Could you check a few things on this model? Use its own coordinates, in mm. A direction names the side the tool comes from. Give positions to 0.01 mm unless a question says otherwise; leave off trailing zeros. Write each loop counter-clockwise with the first axis right and the second up, starting at its lowest first coordinate (ties: lowest second). Pieces come first, ordered by that corner, then holes. Notation, with made-up numbers: (86, -5.5) - (122, -5.5) arc R28 cw to (122, 31.5) - close; hole circle Ø11 at (32, 35). An arc over 180 degrees is marked (long way). Answer as CSV lines item,"result". Start each with the question number.
Q1. If I drill on line 1 along Y through (x, z) = (-65, 2.8); line 2 along Y through (x, z) = (-33.5, 1.8), over which ranges is the centre line in solid material (lowest first)?
Q2. Imagine slicing it at B-B on x = -64. List the corners of the cut face in (y, z) for me.
Q3. Will this pin go through, and if not, where does the flat tip stop? pin 1 Ø1.5 at (y, z) = (-73.5, 1.5) entering from -X.
Q4. We'd pull the mould along X, two halves only. Please class faces 3 (the face through (0, -41, 1)), 4 (the face through (-35.356, -5.994, 1.479)), 5 (the face through (-6.6, -19.1, 0)): pulls with the +X half, pulls with the -X half, needs draft (parallel to the pull), parting line crosses it, or undercut.
Q5. Imagine slicing it at A-A on z = 1.6. List the corners of the cut face in (x, y) for me.
Q6. Imagine slicing it at C-C on y = -52. List the corners of the cut face in (x, z) for me.
Q7. On a 3-axis mill with a long thin cutter (end or side, diameter ignored), from which of +Z, -Z, +X, -X, +Y, -Y can I reach the whole of each face in a straight line? I mean faces 1 (the face through (-65, -10, 1)), 2 (the face through (-6.6, -19.1, 3)). Say none if no direction works.
```python
from build123d import *

# Parameters (mm, degrees)
BOSS_EXTRUDE1_DEPTH = 3


with BuildPart() as part:
    # Sketch1 → Boss-Extrude1 (new body)
    with BuildSketch(Plane.XY):
        with BuildLine():
            Line((0, 0), (-70, 0))
            Line((-70, 0), (-70, -10))
            Line((-70, -10), (-60, -10))
            ThreePointArc((-60, -10), (-35, -5.993420768), (-10, -10))
            ThreePointArc((-10, -10), (-4.161984871, -40), (-10, -70))
            Line((-10, -70), (-10, -80))
            Line((-10, -80), (0, -80))
            Line((0, -80), (0, 0))
        make_face()
    extrude(amount=BOSS_EXTRUDE1_DEPTH)


solid = part.part
```
Conclusion:
1,line 1,"-10 to 0"
1,line 2,"-6.01 to 0"
2,outline,"(-10, 0) - (0, 0) - (0, 3) - (-10, 3) - close"
3,pin 1,"x = -10"
4,face 3,"pulls with the +X half"
4,face 4,"undercut"
4,face 5,"needs draft"
5,outline,"(-70, -10) - (-60, -10) arc R80 cw to (-10, -10) arc R80 cw to (-10, -70) - (-10, -80) - (0, -80) - (0, 0) - (-70, 0) - close"
6,outline,"(-5.07, 0) - (0, 0) - (0, 3) - (-5.07, 3) - close"
7,face 1,"+Z, -Z, -X, -Y"
7,face 2,"+Z, +X, -X, +Y, -Y"
